CAD build for the part. Positions are in the model's coordinates, mm. Give positions to 0.01 mm unless a question says otherwise; leave off trailing zeros. Write each loop counter-clockwise with the first axis right and the second up, starting at its lowest first coordinate (ties: lowest second). Pieces come first, ordered by that corner, then holes. Notation, with made-up numbers: (7, -25) - (32, -25) arc R15 ccw to (32, -18) - close; hole circle Ø10 at (-6, 2). An arc over 180 degrees is marked (long way). Answer as a JSON object with one key per item and string values.
Autodesk Inventor part; units mm, degrees
ref_plane "YZ Plane" through (0, 0, 0) normal (1, 0, 0) x (0, 1, 0)
ref_plane "XZ Plane" through (0, 0, 0) normal (0, 1, 0) x (-1, 0, 0)
ref_plane "XY Plane" through (0, 0, 0) normal (0, 0, 1) x (1, 0, 0)
sketch "Sketch1" plane through (0, 0, 0) normal (0, 0, 1) x (1, 0, 0)
  line L0 (9.2688, 23.2165) -> (-16.1312, 23.2165)
  line L1 (-16.1312, 23.2165) -> (-16.1312, -27.5835)
  line L2 (-16.1312, -27.5835) -> (9.2688, -27.5835)
  line L3 (9.2688, -27.5835) -> (9.2688, 23.2165)
  point P0 (0, 0)
  dimension "d0" = 25.4
  dimension "d1" = 50.8
extrude "Extrusion1" add sketch "Sketch1" along normal blind 5
sketch "Sketch2" plane through (0, 0, 5) normal (0, 0, 1) x (1, 0, 0)
  circle A0 centre (-3.4312, 8.2165) radius 12.3 construction
  circle A1 centre (-3.4312, 8.2165) radius 8.5 construction
  circle A2 centre (-11.9312, 8.2165) radius 1.5
  circle A3 centre (-3.4312, 8.2165) radius 1.5
  circle A4 centre (-3.4312, -0.2835) radius 1.5
  circle A5 centre (5.0688, 8.2165) radius 1.5
  circle A6 centre (-3.4312, 16.7165) radius 1.5
  line L0 (9.2688, 23.2165) -> (-16.1312, 23.2165)
  point P0 (0, 0)
  point P1 (-3.4312, 23.2165)
  dimension "d5" = 17
  dimension "d4" = 24.6
  dimension "d6" = 3
  dimension "d7" = 3
  dimension "d10" = 360
  dimension "d12" = 15
extrude "Extrusion2" cut sketch "Sketch2" against normal up to next
sketch "Sketch3" plane through (-16.1312, -27.5835, 0) normal (-1, 0, 0) x (0, 0, 1)
  line L0 (0, 0) -> (5, 0)
  point P0 (0, 27.5835)
  point P1 (2.5, 2.5)
  point P2 (2.5, 0)
  dimension "d15" = 2.5
hole "Hole1" at (-16.1312, -25.0835, 2.5) direction (1, 0, 0) diameter 2.46 depth 13.6906 tip angle 118
full round fillet "Fillet1" first side at (-16.1312, 7.5235, 2.4506) centre faces at (0.8021, 23.2165, 3.3333) second side at (9.2688, -10.6502, 1.6667)
properties part number "Tilt_Camera_Side_Plate"
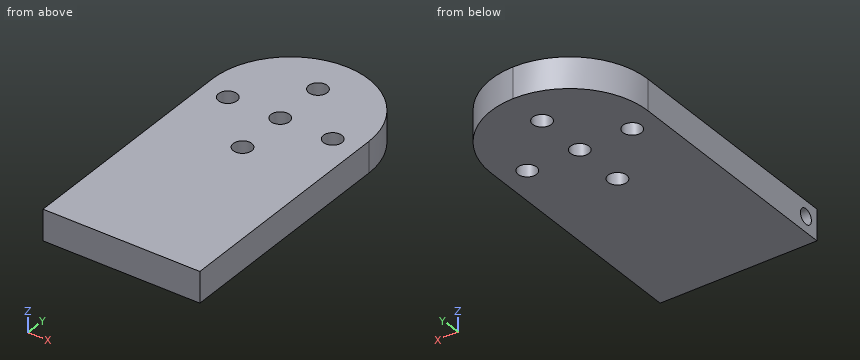
Item 1: Flat gauge pins, fed straight in: P1, Ø1.8, axis at x = -11.93, y = 8.22, coming from the +Z side; P2, Ø1, axis at x = -1, z = 3, coming from the +Y side. Where does each tip first touch, or does it go through?
Entries:
{"P1": "through", "P2": "y = 23.07"}
Item 2: Cut at C-C (z = 3.15). State how many separate pieces and enclosed holes the cut face has, and give its area (3 significant figures).
Entries:
{"separate pieces": "1", "enclosed holes": "5", "area": "1,160 mm2"}
Item 3: Cut at B-B (y = 16). Give the cut face in (x, z), and give its area (3 significant figures).
Entries:
{"outline": "(-14.89, 0) - (-4.75, 0) - (-4.75, 5) - (-14.89, 5) - close; (-2.11, 0) - (8.02, 0) - (8.02, 5) - (-2.11, 5) - close", "area": "101 mm2"}
Item 4: Cut at A-A (y = 0.5). Give the cut face in (x, z).
Entries:
{"outline": "(-16.13, 0) - (-4.71, 0) - (-4.71, 5) - (-16.13, 5) - close; (-2.15, 0) - (9.27, 0) - (9.27, 5) - (-2.15, 5) - close"}
Item 5: Probe line 1 (Y direction, x = -4, z = 2.45); line 2 (Y direction, x = -3.5, z = 1.7); line 3 (Y direction, x = 5.5, z = 4.6). List the from-to ranges inside material, lowest first. Write a range as from..to.
Entries:
{"line 1": "-27.58..-26.31, -23.85..-1.67, 1.1..6.83, 9.6..15.33, 18.1..23.2", "line 2": "-27.58..-26.02, -24.15..-1.78, 1.21..6.72, 9.71..15.22, 18.21..23.22", "line 3": "-27.58..6.78, 9.65..19.55"}
